Print and shaded views of the part. All mm, measured from the part's lowest x, y and z. A direction names the side the tool comes from. Round coordinates to 2 decimals unless told otherwise and drop trailing zeros. Write each loop counter-clockwise with the first axis right and the second up, starting at its lowest first coordinate (ties: lowest second). Pieces come first, ordered by that corner, then holes. Notation, with made-up numbers: (46.5, 20) - (93.5, 20) arc R12 cw to (93.5, 24) - close; hole circle Ø5 at (-14.75, 51.25). An arc over 180 degrees is marked (long way). One line per item, written item: value.
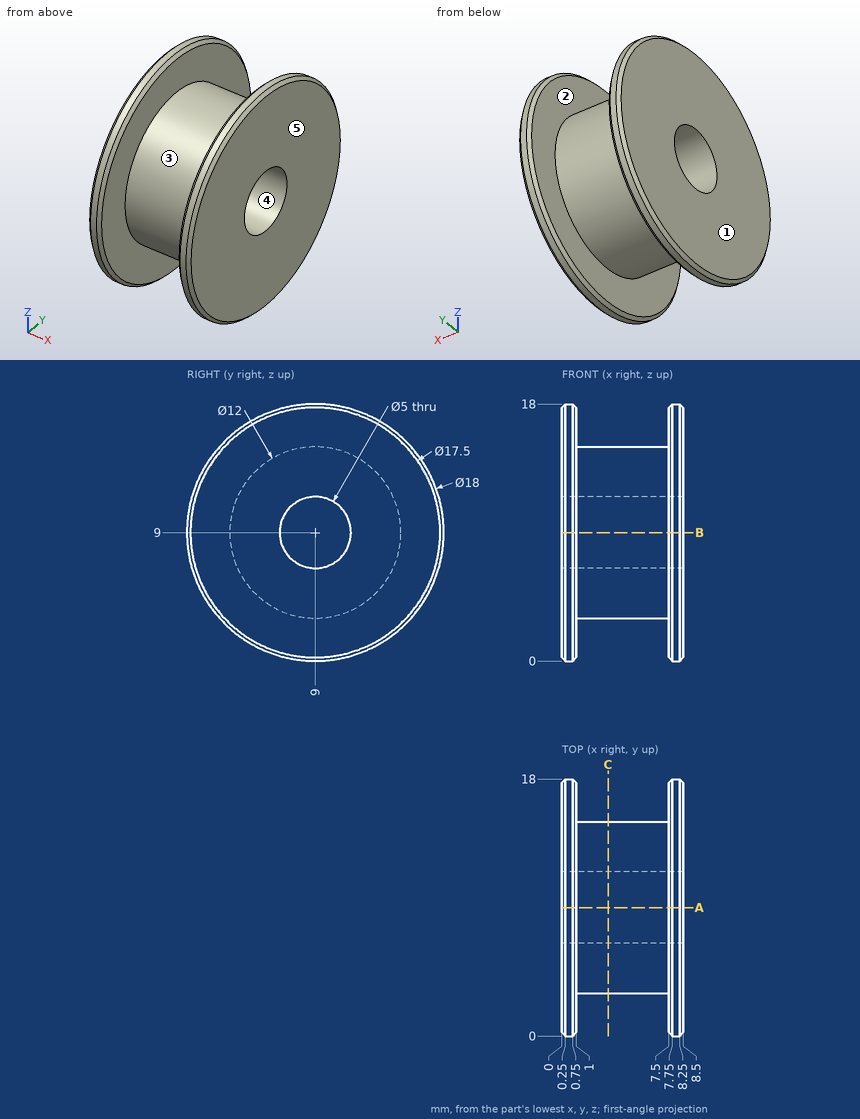
1. Band-saw the part on C-C on x = 3.25. Write the cut outline in (y, z), plus the area to 3 significant figures.
Report:
outline: circle Ø12 at (9, 9); hole circle Ø5 at (9, 9)
area: 93.5 mm²
2. Mould opens along Z. For the marked faces 3, 4 and 5 say: released by +Z, released by -Z, zero draft, split by the parting line, or undercut.
Report:
face 3: split by the parting line
face 4: undercut
face 5: zero draft
3. Tool access for the marked faces 1 and 2: list every direction of +Z, -Z, +X, -X, +Y, -Y with a clear straight run to the whole face (end or side of a thin tool).
Report:
face 1: +Z, -Z, -X, +Y, -Y
face 2: none
4. Band-saw the part on A-A on y = 9. Write the cut outline in (x, z), plus the area to 4 significant figures.
Report:
outline: (0, 0.25) - (0.25, 0) - (0.75, 0) - (1, 0.25) - (1, 3) - (7.5, 3) - (7.5, 0.25) - (7.75, 0) - (8.25, 0) - (8.5, 0.25) - (8.5, 6.5) - (0, 6.5) - close; (0, 11.5) - (8.5, 11.5) - (8.5, 17.75) - (8.25, 18) - (7.75, 18) - (7.5, 17.75) - (7.5, 15) - (1, 15) - (1, 17.75) - (0.75, 18) - (0.25, 18) - (0, 17.75) - close
area: 71.25 mm²
5. Drop flat-ended pins along their axis: pin 1 (5 mm diameter, centred on x = 4, z = 15, fed in from -Y); pin 2 (4.5 mm diameter, centred on y = 9, z = 9, fed in from +X). Give the stop position or say it passes through.
Report:
pin 1: y = 4.13
pin 2: through
6. Wall check: probe 1 along X at (y, z) = (3.25, 11); probe 2 along Z at (x, y) = (4.5, 9); probe 3 along Z at (x, y) = (2, 7.25). Give the ranges that are in metal, low to high. Write a range as [from, to].
Report:
probe 1: [0, 1], [7.5, 8.5]
probe 2: [3, 6.5], [11.5, 15]
probe 3: [3.26, 7.21], [10.79, 14.74]
